Read the model definition and answer for the solid it produces. Units are mm, in the model's axes. Coordinates: 2 decimals unless noted, no trailing zeros. Write each loop counter-clockwise with the first axis right and the second up, starting at its lowest first coordinate (ties: lowest second). Pieces come first, ordered by that corner, then holes.
from build123d import *

# Parameters (mm, degrees)
SKETCH1_W           = 106.68
SKETCH1_H           = 68.58
BOSS_EXTRUDE1_DEPTH = 1.524
CUT_EXTRUDE1_REACH  = 65.429
SKETCH2_R           = 3.175
CUT_EXTRUDE2_REACH  = 65.429
SKETCH3_R           = 4.445
FILLET1_R           = 2.54
CUT_EXTRUDE3_REACH  = 65.429
SKETCH4_R           = 1.0414
SKETCH4_R_2         = 1.0795
CUT_EXTRUDE4_REACH  = 65.429
SKETCH5_R           = 1.016
CUT_EXTRUDE5_REACH  = 65.429


with BuildPart() as part:
    # Sketch1 → Boss-Extrude1 (new body)
    with BuildSketch(Plane.XY):
        Rectangle(SKETCH1_W, SKETCH1_H)
    extrude(amount=BOSS_EXTRUDE1_DEPTH)

    # Sketch2 → Cut-Extrude1 (cut, up to next)
    with BuildSketch(Plane.XY.offset(1.524), mode=Mode.PRIVATE) as cut_extrude1_sk1:
        with Locations((-48.26, 29.21)):
            Circle(SKETCH2_R)
    cut_extrude1_tool1 = extrude(cut_extrude1_sk1.sketch, amount=-CUT_EXTRUDE1_REACH, mode=Mode.PRIVATE) & part.part
    # Sketch2 → Cut-Extrude1 (cut, up to next)
    with BuildSketch(Plane.XY.offset(1.524), mode=Mode.PRIVATE) as cut_extrude1_sk2:
        with Locations((-48.26, -29.21)):
            Circle(SKETCH2_R)
    cut_extrude1_tool2 = extrude(cut_extrude1_sk2.sketch, amount=-CUT_EXTRUDE1_REACH, mode=Mode.PRIVATE) & part.part
    # Sketch2 → Cut-Extrude1 (cut, up to next)
    with BuildSketch(Plane.XY.offset(1.524), mode=Mode.PRIVATE) as cut_extrude1_sk3:
        with Locations((48.26, -29.21)):
            Circle(SKETCH2_R)
    cut_extrude1_tool3 = extrude(cut_extrude1_sk3.sketch, amount=-CUT_EXTRUDE1_REACH, mode=Mode.PRIVATE) & part.part
    # Sketch2 → Cut-Extrude1 (cut, up to next)
    with BuildSketch(Plane.XY.offset(1.524), mode=Mode.PRIVATE) as cut_extrude1_sk4:
        with Locations((48.26, 29.21)):
            Circle(SKETCH2_R)
    cut_extrude1_tool4 = extrude(cut_extrude1_sk4.sketch, amount=-CUT_EXTRUDE1_REACH, mode=Mode.PRIVATE) & part.part
    add(cut_extrude1_tool1.solids().sort_by_distance((-48.26, 29.21, 1.524))[0], mode=Mode.SUBTRACT)
    add(cut_extrude1_tool2.solids().sort_by_distance((-48.26, -29.21, 1.524))[0], mode=Mode.SUBTRACT)
    add(cut_extrude1_tool3.solids().sort_by_distance((48.26, -29.21, 1.524))[0], mode=Mode.SUBTRACT)
    add(cut_extrude1_tool4.solids().sort_by_distance((48.26, 29.21, 1.524))[0], mode=Mode.SUBTRACT)

    # Sketch3 → Cut-Extrude2 (cut, up to next)
    with BuildSketch(Plane.XY.offset(1.524), mode=Mode.PRIVATE) as cut_extrude2_sk1:
        with Locations((34.798, -25.4)):
            Circle(SKETCH3_R)
    cut_extrude2_tool1 = extrude(cut_extrude2_sk1.sketch, amount=-CUT_EXTRUDE2_REACH, mode=Mode.PRIVATE) & part.part
    # Sketch3 → Cut-Extrude2 (cut, up to next)
    with BuildSketch(Plane.XY.offset(1.524), mode=Mode.PRIVATE) as cut_extrude2_sk2:
        with Locations((34.798, -8.89)):
            Circle(SKETCH3_R)
    cut_extrude2_tool2 = extrude(cut_extrude2_sk2.sketch, amount=-CUT_EXTRUDE2_REACH, mode=Mode.PRIVATE) & part.part
    # Sketch3 → Cut-Extrude2 (cut, up to next)
    with BuildSketch(Plane.XY.offset(1.524), mode=Mode.PRIVATE) as cut_extrude2_sk3:
        with Locations((34.798, 8.89)):
            Circle(SKETCH3_R)
    cut_extrude2_tool3 = extrude(cut_extrude2_sk3.sketch, amount=-CUT_EXTRUDE2_REACH, mode=Mode.PRIVATE) & part.part
    # Sketch3 → Cut-Extrude2 (cut, up to next)
    with BuildSketch(Plane.XY.offset(1.524), mode=Mode.PRIVATE) as cut_extrude2_sk4:
        with Locations((34.798, 25.4)):
            Circle(SKETCH3_R)
    cut_extrude2_tool4 = extrude(cut_extrude2_sk4.sketch, amount=-CUT_EXTRUDE2_REACH, mode=Mode.PRIVATE) & part.part
    add(cut_extrude2_tool1.solids().sort_by_distance((34.798, -25.4, 1.524))[0], mode=Mode.SUBTRACT)
    add(cut_extrude2_tool2.solids().sort_by_distance((34.798, -8.89, 1.524))[0], mode=Mode.SUBTRACT)
    add(cut_extrude2_tool3.solids().sort_by_distance((34.798, 8.89, 1.524))[0], mode=Mode.SUBTRACT)
    add(cut_extrude2_tool4.solids().sort_by_distance((34.798, 25.4, 1.524))[0], mode=Mode.SUBTRACT)

    # Fillet1
    fillet1_edges = [part.edges().sort_by_distance(p)[0] for p in [
        (53.34, -34.29, 0.762),
        (-53.34, -34.29, 0.762),
        (-53.34, 34.29, 0.762),
        (53.34, 34.29, 0.762),
    ]]
    fillet(fillet1_edges, radius=FILLET1_R)

    # Sketch4 → Cut-Extrude3 (cut, up to next)
    with BuildSketch(Plane.XY.offset(1.524), mode=Mode.PRIVATE) as cut_extrude3_sk1:
        with Locations((-23.241, -26.0096)):
            Circle(SKETCH4_R)
    cut_extrude3_tool1 = extrude(cut_extrude3_sk1.sketch, amount=-CUT_EXTRUDE3_REACH, mode=Mode.PRIVATE) & part.part
    # Sketch4 → Cut-Extrude3 (cut, up to next)
    with BuildSketch(Plane.XY.offset(1.524), mode=Mode.PRIVATE) as cut_extrude3_sk2:
        with Locations((-33.274, -26.0096)):
            Circle(SKETCH4_R)
    cut_extrude3_tool2 = extrude(cut_extrude3_sk2.sketch, amount=-CUT_EXTRUDE3_REACH, mode=Mode.PRIVATE) & part.part
    # Sketch4 → Cut-Extrude3 (cut, up to next)
    with BuildSketch(Plane.XY.offset(1.524), mode=Mode.PRIVATE) as cut_extrude3_sk3:
        with Locations((-28.2448, 25.908)):
            Circle(SKETCH4_R)
    cut_extrude3_tool3 = extrude(cut_extrude3_sk3.sketch, amount=-CUT_EXTRUDE3_REACH, mode=Mode.PRIVATE) & part.part
    # Sketch4 → Cut-Extrude3 (cut, up to next)
    with BuildSketch(Plane.XY.offset(1.524), mode=Mode.PRIVATE) as cut_extrude3_sk4:
        with Locations((46.609, 19.558)):
            Circle(SKETCH4_R_2)
    cut_extrude3_tool4 = extrude(cut_extrude3_sk4.sketch, amount=-CUT_EXTRUDE3_REACH, mode=Mode.PRIVATE) & part.part
    # Sketch4 → Cut-Extrude3 (cut, up to next)
    with BuildSketch(Plane.XY.offset(1.524), mode=Mode.PRIVATE) as cut_extrude3_sk5:
        with Locations((46.609, -14.605)):
            Circle(SKETCH4_R_2)
    cut_extrude3_tool5 = extrude(cut_extrude3_sk5.sketch, amount=-CUT_EXTRUDE3_REACH, mode=Mode.PRIVATE) & part.part
    add(cut_extrude3_tool1.solids().sort_by_distance((-23.241, -26.0096, 1.524))[0], mode=Mode.SUBTRACT)
    add(cut_extrude3_tool2.solids().sort_by_distance((-33.274, -26.0096, 1.524))[0], mode=Mode.SUBTRACT)
    add(cut_extrude3_tool3.solids().sort_by_distance((-28.2448, 25.908, 1.524))[0], mode=Mode.SUBTRACT)
    add(cut_extrude3_tool4.solids().sort_by_distance((46.609, 19.558, 1.524))[0], mode=Mode.SUBTRACT)
    add(cut_extrude3_tool5.solids().sort_by_distance((46.609, -14.605, 1.524))[0], mode=Mode.SUBTRACT)

    # Sketch5 → Cut-Extrude4 (cut, up to next)
    with BuildSketch(Plane.XY.offset(1.524), mode=Mode.PRIVATE) as cut_extrude4_sk1:
        with Locations((-43.942, 0)):
            Circle(SKETCH5_R)
    cut_extrude4_tool1 = extrude(cut_extrude4_sk1.sketch, amount=-CUT_EXTRUDE4_REACH, mode=Mode.PRIVATE) & part.part
    add(cut_extrude4_tool1.solids().sort_by_distance((-43.942, 0, 1.524))[0], mode=Mode.SUBTRACT)

    # Sketch6 → Cut-Extrude5 (cut, up to next)
    with BuildSketch(Plane.XY.offset(1.524), mode=Mode.PRIVATE) as cut_extrude5_sk1:
        with BuildLine():
            Line((-44.7548, 16.129), (-44.7548, 14.1732))
            ThreePointArc((-44.7548, 14.1732), (-45.3898, 13.5382), (-46.0248, 14.1732))
            Line((-46.0248, 14.1732), (-46.0248, 16.129))
            ThreePointArc((-46.0248, 16.129), (-45.3898, 16.764), (-44.7548, 16.129))
        make_face()
    cut_extrude5_tool1 = extrude(cut_extrude5_sk1.sketch, amount=-CUT_EXTRUDE5_REACH, mode=Mode.PRIVATE) & part.part
    # Sketch6 → Cut-Extrude5 (cut, up to next)
    with BuildSketch(Plane.XY.offset(1.524), mode=Mode.PRIVATE) as cut_extrude5_sk2:
        with BuildLine():
            Line((-44.7548, -14.3002), (-44.7548, -16.256))
            ThreePointArc((-44.7548, -16.256), (-45.3898, -16.891), (-46.0248, -16.256))
            Line((-46.0248, -16.256), (-46.0248, -14.3002))
            ThreePointArc((-46.0248, -14.3002), (-45.3898, -13.6652), (-44.7548, -14.3002))
        make_face()
    cut_extrude5_tool2 = extrude(cut_extrude5_sk2.sketch, amount=-CUT_EXTRUDE5_REACH, mode=Mode.PRIVATE) & part.part
    add(cut_extrude5_tool1.solids().sort_by_distance((-45.3898, 15.1511, 1.524))[0], mode=Mode.SUBTRACT)
    add(cut_extrude5_tool2.solids().sort_by_distance((-45.3898, -15.2781, 1.524))[0], mode=Mode.SUBTRACT)


solid = part.part
Item 1: The part is cut by section A-A (y = 8.89). Give the vertices of the cut face in (x, z).
Item 2: Determine the mould class of faces 1 (the cylindrical face through (52.576, 33.566, 0.773)), 2 (the flat face through (-1, 0, 1.524)), 3 (the cylindrical face through (30.357, 25.595, 0.773)) for opening direction X: +X half, -X half, draft (parallel to the pull), parting line (faces both ways), or undercut.
Item 3: Find the intervals of material crossed by probe 1 along Y at (x, z) = (48.26, 1.05) (3 decimals); probe 2 along X at (y, z) = (-31, 1.4); probe 3 along X at (y, z) = (19.5, 0.15), in increasing order.
Item 4: The part is cut by section B-B (z = 0.8). State how many separate pieces and enclosed holes the cut face has, and give its area (3 significant figures).
Item 5: The part is cut by section C-C (x = 35). Give the vertices of the cut face in (y, z).
Item 6: Given pin 1 (7.5 mm diameter, centred on x = 48.26, y = -29.21, fed in from -Z), flat-ended and moving along its own axis, determine where the tip first touches the part or whether it passes through.
Answer:
1. outline: (-53.34, 0) - (30.35, 0) - (30.35, 1.52) - (-53.34, 1.52) - close; (39.24, 0) - (53.34, 0) - (53.34, 1.52) - (39.24, 1.52) - close
2. face 1: +X half
2. face 2: draft
2. face 3: undercut
3. probe 1: y = -34.29 to -32.385, -26.035 to 26.035, 32.385 to 34.29
3. probe 2: x = -53.34 to -50.88, -45.64 to 45.64, 50.88 to 53.34
3. probe 3: x = -53.34 to 45.53, 47.69 to 53.34
4. separate pieces: 1
4. enclosed holes: 16
4. area: 6,910 mm2
5. outline: (-34.29, 0) - (-29.84, 0) - (-29.84, 1.52) - (-34.29, 1.52) - close; (-20.96, 0) - (-13.33, 0) - (-13.33, 1.52) - (-20.96, 1.52) - close; (-4.45, 0) - (4.45, 0) - (4.45, 1.52) - (-4.45, 1.52) - close; (13.33, 0) - (20.96, 0) - (20.96, 1.52) - (13.33, 1.52) - close; (29.84, 0) - (34.29, 0) - (34.29, 1.52) - (29.84, 1.52) - close
6. pin 1: stops at z = 0
